The figure shows three views and two pictorial views of one solid part (mm, origin at its lowest corner). Answer the questions. A direction names the side the tool comes from. Round coordinates to 2 decimals unless told otherwise and drop trailing zeros. Order: outer loops, then holes, each group sorted by start corner. A loop starts at its lowest first (then second) coordinate and runs counter-clockwise, first axis right, second up. Notation, with made-up numbers: (70.25, 41.25) - (109.25, 41.25) arc R19 cw to (109.25, 71.25) - close; hole circle Ø7 at (74.25, 57). An arc over 180 degrees is marked (long way). Answer as a JSON object with one key per item and string values. Group by question number.
Q1. A cutting plane is placed at B-B on z = 39.5. Determine the outline of the cut face in (x, y) (1 decimal).
Q2. A tool of negligible diameter and unlimited length cuts with its end or side. For the marked faces 4 and 5, from which of +Z, -Z, +X, -X, +Y, -Y can it reach the whole face along a straight path? Write none if from no direction.
Q3. The mould has two halves that part along X. Classify the marked faces 1, 2 and 3: pulls with the +X half, pulls with the -X half, needs draft (parallel to the pull), parting line crosses it, or undercut.
Q4. A cutting plane is placed at C-C on y = 46. Determine the outline of the cut face in (x, z) (1 decimal), and give its area (3 significant figures).
Q5. Consider line 1 (X direction, y = 17.5, z = 19.5) (1 decimal); line 2 (Y direction, x = 25, z = 16); line 3 (X direction, y = 42, z = 39.5) (1 decimal). Determine where each line is inside the solid, lowest interval first.
Q6. A cutting plane is placed at A-A on x = 85. Determine the outline of the cut face in (y, z).
Q7. A cutting plane is placed at D-D on y = 30.5. Determine the outline of the cut face in (x, z) (1 decimal), and give its area (3 significant figures).
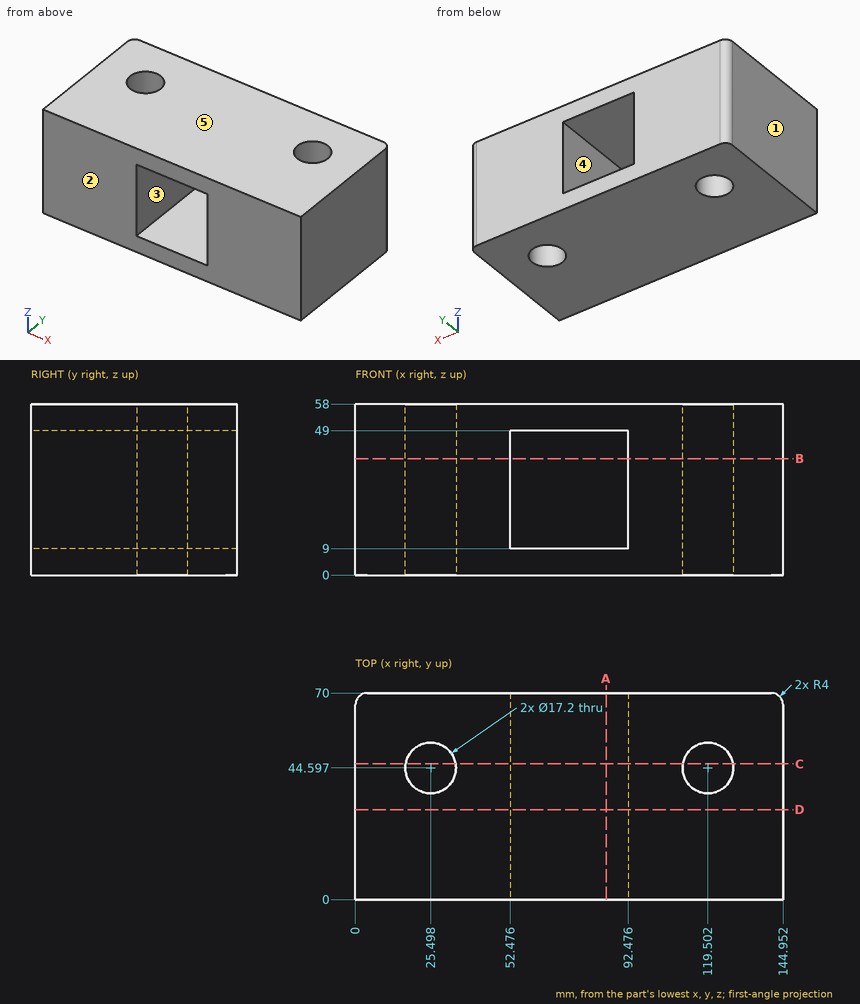
Result set:
{
 "1": {"outline": "(0, 0) - (52.5, 0) - (52.5, 70) - (4, 70) arc R4 ccw to (0, 66) - close; (92.5, 0) - (145, 0) - (145, 66) arc R4 ccw to (141, 70) - (92.5, 70) - close; hole circle Ø17.2 at (25.5, 44.6); hole circle Ø17.2 at (119.5, 44.6)"},
 "2": {"face 4": "+Y, -Y", "face 5": "+Z, +X, -X, +Y, -Y"},
 "3": {"face 1": "pulls with the -X half", "face 2": "needs draft", "face 3": "undercut"},
 "4": {"outline": "(0, 0) - (17, 0) - (17, 58) - (0, 58) - close; (34, 0) - (111, 0) - (111, 58) - (34, 58) - close; (128, 0) - (145, 0) - (145, 58) - (128, 58) - close; hole (52.5, 9) - (92.5, 9) - (92.5, 49) - (52.5, 49) - close", "area": "4,840 mm²"},
 "5": {"line 1": "x = 0 to 52.5, 92.5 to 145", "line 2": "y = 0 to 36.01, 53.18 to 70", "line 3": "x = 0 to 17.3, 33.7 to 52.5, 92.5 to 111.3, 127.7 to 145"},
 "6": {"outline": "(0, 0) - (70, 0) - (70, 9) - (0, 9) - close; (0, 49) - (70, 49) - (70, 58) - (0, 58) - close"},
 "7": {"outline": "(0, 0) - (145, 0) - (145, 58) - (0, 58) - close; hole (52.5, 9) - (92.5, 9) - (92.5, 49) - (52.5, 49) - close", "area": "6,810 mm²"}
}
